Check sheet for the modelled part. Datum: model origin and axes. Units: mm. Face numbers are marked on the shaded views. A direction names the side the tool comes from. Round coordinates to 2 decimals unless told otherwise and drop trailing zeros. Loops run counter-clockwise (first coordinate to the right, second up) from the corner with the lowest first, then second, coordinate; pieces in that order, holes last. Notation, with made-up numbers: (45, 23) -> (82, 23) arc R16 ccw to (82, 53) -> close; hole circle Ø4 at (-31, 79.25). An arc over 180 degrees is marked (long way). One line per question, with ' | ' between items.
```python
from build123d import *

# Parameters (mm, degrees)
EXTRUDE_1_DEPTH = 4
EXTRUDE_2_DEPTH = 20
FILLET_1_R      = 0.5
FILLET_2_R      = 0.5


with BuildPart() as part:
    # 草图1 → 凸台-拉伸1 (new body)
    with BuildSketch(Plane(origin=(0, 0, 0), x_dir=(1, 0, 0), z_dir=(0, 1, 0))):
        with BuildLine():
            Line((-10, -20), (10, -20))
            ThreePointArc((10, -20), (17.071067812, -17.071067812), (20, -10))
            Line((20, -10), (20, 10))
            ThreePointArc((20, 10), (17.071067812, 17.071067812), (10, 20))
            Line((10, 20), (-10, 20))
            ThreePointArc((-10, 20), (-17.071067812, 17.071067812), (-20, 10))
            Line((-20, 10), (-20, -10))
            ThreePointArc((-20, -10), (-17.071067812, -17.071067812), (-10, -20))
        make_face()
        Polygon((-10, 3.960573477), (-15, 3.960573477), (-15, 15), (15, 15), (15, -15), (-15, -15), (-15, -3.960573477), (-10, -3.960573477), (-10, -10), (10, -10), (10, 10), (-10, 10), align=None, mode=Mode.SUBTRACT)
    extrude(amount=EXTRUDE_1_DEPTH)

    # 草图2 → 凸台-拉伸2 (add)
    with BuildSketch(Plane.ZY.offset(10)):
        Polygon((-10, 4), (10, 4), (10, 4.5), (2.5, 4.5), (2.5, 5.5), (-2.5, 5.5), (-2.5, 4.5), (-10, 4.5), align=None)
    extrude(amount=-EXTRUDE_2_DEPTH)

    # 圆角1
    fillet_1_edges = [part.edges().sort_by_distance(p)[0] for p in [
        (10, 4.5, -6.25),
        (0, 4.5, -10),
        (10, 5, -2.5),
        (0, 4.5, -2.5),
        (10, 5, 2.5),
        (10, 4.5, 6.25),
        (0, 4.5, 2.5),
        (0, 4.5, 10),
        (-10, 4.5, 6.25),
        (-10, 5, 2.5),
        (-10, 5, -2.5),
        (-10, 4.5, -6.25),
    ]]
    fillet(fillet_1_edges, radius=FILLET_1_R - 0.0001)  # a hair under: the kernel refuses the full size

    # 圆角2
    fillet_2_edges = [part.edges().sort_by_distance(p)[0] for p in [
        (9.85358268, 5.5, 2.35358268),
        (0, 5.5, 2.5),
        (-9.85358268, 5.5, 2.35358268),
        (-10, 5.5, 0),
        (-9.85358268, 5.5, -2.35358268),
        (0, 5.5, -2.5),
        (9.85358268, 5.5, -2.35358268),
        (10, 5.5, 0),
    ]]
    fillet(fillet_2_edges, radius=FILLET_2_R - 0.0001)  # a hair under: the kernel refuses the full size


solid = part.part
```
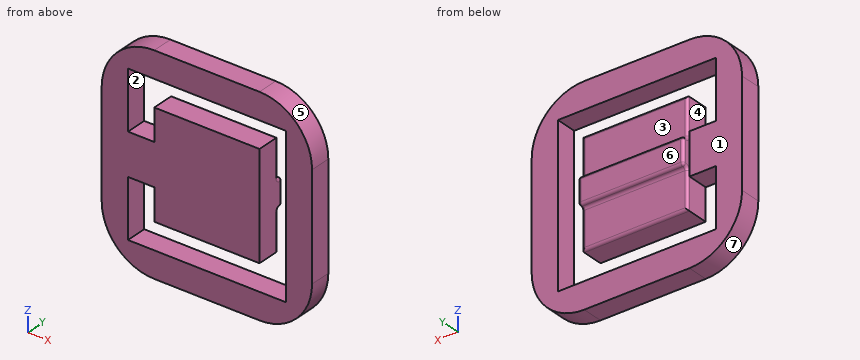
(1) Mould release check, pull along Z, two halves, no side actions. Record for the marked faces 4, 5, 6 and 7: +Z half, -Z half, draft (parallel to the pull), parting line (faces both ways), or undercut.
Answer:
face 4: undercut | face 5: +Z half | face 6: draft | face 7: -Z half
(2) Sectioned sample at D-D, the plane z = 0.5. Record the cut outline in (x, y), and give its area (3 significant figures).
Answer:
outline: (-20, 0) -> (10, 0) -> (10, 5) arc R0.5 ccw to (9.5, 5.5) -> (-9.5, 5.5) arc R0.5 ccw to (-10, 5) -> (-10, 4) -> (-20, 4) -> close; (15, 0) -> (20, 0) -> (20, 4) -> (15, 4) -> close | area: 170 mm2
(3) Set-up check for the marked faces 1, 2 and 3: record each of +Z, -Z, +X, -X, +Y, -Y from which the full face is reachable in a straight line by a thin tool's end or side.
Answer:
face 1: +Y | face 2: +Y, -Y | face 3: +Z, +X, -X, +Y
(4) Scan lines: probe 1 along X at (y, z) = (0.75, -5.5); probe 2 along Z at (x, y) = (-12.5, 1.05). Record each from-to range of solid material in increasing order.
Answer:
probe 1: x = -20 to -15, -10 to 10, 15 to 20 | probe 2: z = -19.68 to -15, -3.96 to 3.96, 15 to 19.68
(5) Sectioned sample at C-C, the plane y = 2.9. Record the cut outline in (x, z).
Answer:
outline: (-20, -10) arc R10 ccw to (-10, -20) -> (10, -20) arc R10 ccw to (20, -10) -> (20, 10) arc R10 ccw to (10, 20) -> (-10, 20) arc R10 ccw to (-20, 10) -> close; hole (-15, -15) -> (15, -15) -> (15, 15) -> (-15, 15) -> (-15, 3.96) -> (-10, 3.96) -> (-10, 10) -> (10, 10) -> (10, -10) -> (-10, -10) -> (-10, -3.96) -> (-15, -3.96) -> close
(6) Go/stop test with flat-tipped pins: pin 1 (2 mm diameter, centred on x = 0, z = -5, fed in from +Y); pin 2 (1.2 mm diameter, centred on x = -13, y = 1, fed in from +Z); pin 3 (4 mm diameter, centred on x = -14, z = -13.5, fed in from +Y). Record where each tip stops, or that it passes through.
Answer:
pin 1: stops at y = 4.5 | pin 2: stops at z = 19.71 | pin 3: stops at y = 4
(7) Sectioned sample at A-A, the plane z = -6.5. Record the cut outline in (x, y).
Answer:
outline: (-20, 0) -> (-15, 0) -> (-15, 4) -> (-20, 4) -> close; (-10, 0) -> (10, 0) -> (10, 4) arc R0.5 ccw to (9.5, 4.5) -> (-9.5, 4.5) arc R0.5 ccw to (-10, 4) -> close; (15, 0) -> (20, 0) -> (20, 4) -> (15, 4) -> close
(8) Sectioned sample at B-B, the plane x = -7.5. Count the separate pieces of the cut face and the enclosed holes in it, and give its area (3 significant figures).
Answer:
separate pieces: 3 | enclosed holes: 0 | area: 135 mm2
